```python
from build123d import *

# Parameters (mm, degrees)
SKETCH_1_W          = 25
SKETCH_1_H          = 25
EXTRUDE_1_DEPTH     = 3
SKETCH_2_W          = 3
SKETCH_2_H          = 100
EXTRUDE_2_DEPTH     = 190
FILLET_1_R          = 10
SKETCH_3_W          = 20
SKETCH_3_H          = 15
CUT_EXTRUDE_2_DEPTH = 10
FILLET_2_R          = 10
FILLET_3_R          = 10


with BuildPart() as part:
    # 草图1 → 凸台-拉伸1 (new body)
    with BuildSketch(Plane.XY):
        with Locations((-100.141216583, -61.148491789)):
            Rectangle(SKETCH_1_W, SKETCH_1_H)
    extrude(amount=EXTRUDE_1_DEPTH)

    # 草图2 → 凸台-拉伸2 (add)
    with BuildSketch(Plane.XY.offset(3)):
        with Locations((-89.141216583, -23.452816851)):
            Rectangle(SKETCH_2_W, SKETCH_2_H)
    extrude(amount=EXTRUDE_2_DEPTH)

    # 圆角1
    fillet_1_edges = [part.edges().sort_by_distance(p)[0] for p in [
        (-90.641216583, -61.05065432, 3),
    ]]
    fillet(fillet_1_edges, radius=FILLET_1_R)

    # 草图3 → 切除-拉伸2 (cut)
    with BuildSketch(Plane(origin=(-87.641216583, 0, 0), x_dir=(0, 0, -1), z_dir=(1, 0, 0))):
        with Locations((-25, 4.047183149)):
            Rectangle(SKETCH_3_W, SKETCH_3_H)
        with Locations((-55, 4.047183149)):
            Rectangle(SKETCH_3_W, SKETCH_3_H)
        with Locations((-85, 4.047183149)):
            Rectangle(SKETCH_3_W, SKETCH_3_H)
        with Locations((-115, 4.047183149)):
            Rectangle(SKETCH_3_W, SKETCH_3_H)
        with Locations((-145, 4.047183149)):
            Rectangle(SKETCH_3_W, SKETCH_3_H)
        with Locations((-175, 4.047183149)):
            Rectangle(SKETCH_3_W, SKETCH_3_H)
        with Locations((-55, -22.952816851)):
            Rectangle(SKETCH_3_W, SKETCH_3_H)
        with Locations((-85, -22.952816851)):
            Rectangle(SKETCH_3_W, SKETCH_3_H)
        with Locations((-115, -22.952816851)):
            Rectangle(SKETCH_3_W, SKETCH_3_H)
        with Locations((-145, -22.952816851)):
            Rectangle(SKETCH_3_W, SKETCH_3_H)
        with Locations((-175, -22.952816851)):
            Rectangle(SKETCH_3_W, SKETCH_3_H)
        with Locations((-55, -49.952816851)):
            Rectangle(SKETCH_3_W, SKETCH_3_H)
        with Locations((-85, -49.952816851)):
            Rectangle(SKETCH_3_W, SKETCH_3_H)
        with Locations((-115, -49.952816851)):
            Rectangle(SKETCH_3_W, SKETCH_3_H)
        with Locations((-145, -49.952816851)):
            Rectangle(SKETCH_3_W, SKETCH_3_H)
        with Locations((-175, -49.952816851)):
            Rectangle(SKETCH_3_W, SKETCH_3_H)
        with Locations((-25, -22.952816851)):
            Rectangle(SKETCH_3_W, SKETCH_3_H)
        with Locations((-25, -49.952816851)):
            Rectangle(SKETCH_3_W, SKETCH_3_H)
    extrude(amount=-CUT_EXTRUDE_2_DEPTH, mode=Mode.SUBTRACT)

    # 圆角2
    fillet_2_edges = [part.edges().sort_by_distance(p)[0] for p in [
        (-89.141216583, 26.547183149, 193),
    ]]
    fillet(fillet_2_edges, radius=FILLET_2_R)

    # 圆角3
    fillet_3_edges = [part.edges().sort_by_distance(p)[0] for p in [
        (-89.141216583, 26.547183149, 3),
    ]]
    fillet(fillet_3_edges, radius=FILLET_3_R)


solid = part.part
```
The listing builds one solid part. Answer for the finished solid, in the listing's coordinates (mm). A direction names the side the tool comes from. Coordinates: 2 decimals unless noted, no trailing zeros. Write each loop counter-clockwise with the first axis right and the second up, starting at its lowest first coordinate (ties: lowest second). Pieces come first, ordered by that corner, then holes. Notation, with made-up numbers: (10, 13.25) - (26, 13.25) arc R26 ccw to (26, 34.25) - close; hole circle Ø8 at (36, 69). An arc over 180 degrees is marked (long way). Return JSON: item names as keys, results as strings. Group by question number.
Q1. Flat-ended cylindrical pins translate along their axes: pin 1 Ø10 at (y, z) = (-21, 159) entering from -X; pin 2 Ø2.5 at (x, z) = (-89, 25.5) entering from -Y; pin 3 Ø1.5 at (x, y) = (-88.5, 0.5) entering from -Z. Find the tip coordinate at first contact, or state that the pin passes through.
Q2. Which of the six approach directions +Z, -Z, +X, -X, +Y, -Y give full straight-line access (tool end or side, diameter ignored) to faces 1 (the cylindrical face through (-89.12, 23.54, 190.15)), 2 (the flat face through (-89, -73.453, 91)), 3 (the flat face through (-90.641, -24, 97))?
Q3. The part is cut by section D-D on y = -64.5. Write down the section's boundary in (x, z).
Q4. The part is cut by section C-C on x = -105.25. Write down the section's boundary in (y, z), and give its area (3 significant figures).
Q5. The part is cut by section B-B on y = -22.5. Write down the section's boundary in (x, z), and give its area (3 significant figures).
Q6. Find the intervals of material crossed by line 1 along Y through (x, z) = (-90.25, 33); line 2 along X through (y, z) = (-58, 166); line 3 along Y through (x, z) = (-90, 126.5), in increasing order. Write a range as [from, to].
Q7. The part is cut by section A-A on z = 78.5. Write down the section's boundary in (x, y), and give its area (3 significant figures).
Evaluation:
{
 "1": {"pin 1": "stops at x = -90.64", "pin 2": "stops at y = -73.45", "pin 3": "stops at z = 3"},
 "2": {"face 1": "+Z, +X, -X, +Y", "face 2": "+Z, +X, -X, -Y", "face 3": "+Z, -X, +Y"},
 "3": {"outline": "(-112.64, 0) - (-87.64, 0) - (-87.64, 193) - (-90.64, 193) - (-90.64, 13) arc R10 cw to (-100.64, 3) - (-112.64, 3) - close"},
 "4": {"outline": "(-73.65, 0) - (-48.65, 0) - (-48.65, 3) - (-73.65, 3) - close", "area": "75.0 mm2"},
 "5": {"outline": "(-90.64, 3) - (-87.64, 3) - (-87.64, 15) - (-90.64, 15) - close; (-90.64, 35) - (-87.64, 35) - (-87.64, 45) - (-90.64, 45) - close; (-90.64, 65) - (-87.64, 65) - (-87.64, 75) - (-90.64, 75) - close; (-90.64, 95) - (-87.64, 95) - (-87.64, 105) - (-90.64, 105) - close; (-90.64, 125) - (-87.64, 125) - (-87.64, 135) - (-90.64, 135) - close; (-90.64, 155) - (-87.64, 155) - (-87.64, 165) - (-90.64, 165) - close; (-90.64, 185) - (-87.64, 185) - (-87.64, 193) - (-90.64, 193) - close", "area": "210 mm2"},
 "6": {"line 1": "y = [-73.45, -57.45], [-42.45, -30.45], [-15.45, -3.45], [11.55, 26.55]", "line 2": "x = [-90.64, -87.64]", "line 3": "y = [-73.45, 26.55]"},
 "7": {"outline": "(-90.64, -73.45) - (-87.64, -73.45) - (-87.64, -57.45) - (-90.64, -57.45) - close; (-90.64, -42.45) - (-87.64, -42.45) - (-87.64, -30.45) - (-90.64, -30.45) - close; (-90.64, -15.45) - (-87.64, -15.45) - (-87.64, -3.45) - (-90.64, -3.45) - close; (-90.64, 11.55) - (-87.64, 11.55) - (-87.64, 26.55) - (-90.64, 26.55) - close", "area": "165 mm2"}
}
